Part model, mm, in its own coordinate system. Face numbers are marked on the shaded views. A direction names the side the tool comes from. Give positions to 0.01 mm unless a question says otherwise; leave off trailing zeros. Write each loop counter-clockwise with the first axis right and the second up, starting at its lowest first coordinate (ties: lowest second). Pieces come first, ordered by that corner, then holes. Notation, with made-up numbers: (89, 64.5) - (148, 64.5) arc R34 ccw to (148, 98.5) - close; hole circle Ø8 at (24, 34). An arc over 180 degrees is marked (long way). Answer as a JSON object with one key per item and string values. Group by question number.
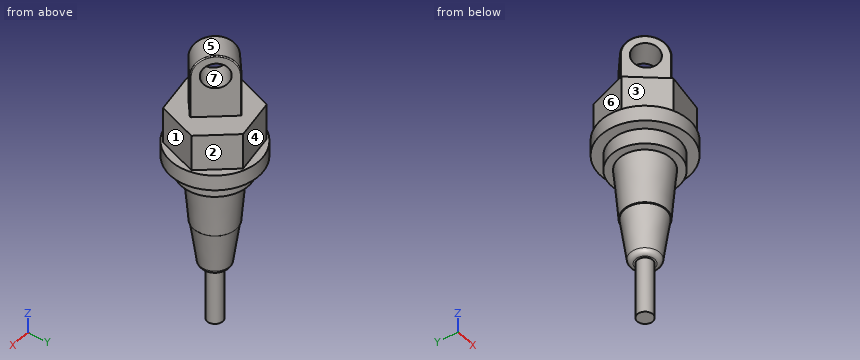
```python
from build123d import *

# Parameters (mm, degrees)
SKETCH_1_R      = 8.5
EXTRUDE_1_DEPTH = 3
EXTRUDE_2_DEPTH = 7
SKETCH_3_R      = 6.5
EXTRUDE_3_DEPTH = 3
SKETCH_4_R      = 5
EXTRUDE_4_DEPTH = 10
EXTRUDE_4_TAPER = 5
SKETCH_5_R      = 4
EXTRUDE_5_DEPTH = 9
EXTRUDE_5_TAPER = 8
FILLET_1_R      = 0.1
FILLET_2_R      = 1
SKETCH_7_R      = 2.5
EXTRUDE_6_DEPTH = 2.5
FILLET_3_R      = 0.2
SKETCH_8_R      = 1.5
EXTRUDE_7_DEPTH = 11


with BuildPart() as part:
    # 草图1 → 凸台-拉伸1 (new body)
    with BuildSketch(Plane.XY):
        with Locations((0, 6.282173928)):
            Circle(SKETCH_1_R)
    extrude(amount=EXTRUDE_1_DEPTH)

    # 草图2 → 凸台-拉伸2 (add)
    with BuildSketch(Plane.XY.offset(3)):
        Polygon((5.281387937, 0.163328057), (7.939769935, 7.796567113), (2.658381997, 13.915412984), (-5.281387937, 12.401019799), (-7.939769935, 4.767780743), (-2.658381997, -1.351065128), align=None)
    extrude(amount=EXTRUDE_2_DEPTH)

    # 草图3 → 凸台-拉伸3 (add)
    with BuildSketch(Plane(origin=(0, 0, 0), x_dir=(-1, 0, 0), z_dir=(0, 0, -1))):
        with Locations(Location((0, 6.282173928, 0), (0, 0, 180))):
            Circle(SKETCH_3_R)
    extrude(amount=EXTRUDE_3_DEPTH)

    # 草图4 → 凸台-拉伸4 (add)
    with BuildSketch(Plane(origin=(0, 0, -3), x_dir=(-1, 0, 0), z_dir=(0, 0, -1))):
        with Locations((0, 6.282173928)):
            Circle(SKETCH_4_R)
    extrude(amount=EXTRUDE_4_DEPTH, taper=EXTRUDE_4_TAPER)

    # 草图5 → 凸台-拉伸5 (add)
    with BuildSketch(Plane(origin=(0, 0, -13), x_dir=(-1, 0, 0), z_dir=(0, 0, -1))):
        with Locations((0, 6.282173928)):
            Circle(SKETCH_5_R)
    extrude(amount=EXTRUDE_5_DEPTH, taper=EXTRUDE_5_TAPER)

    # 圆角1
    fillet_1_edges = [part.edges().sort_by_distance(p)[0] for p in [
        (4.125113365, 6.282173928, -13),
    ]]
    fillet(fillet_1_edges, radius=FILLET_1_R)

    # 圆角2
    fillet_2_edges = [part.edges().sort_by_distance(p)[0] for p in [
        (2.735132488, 6.282173928, -22),
    ]]
    fillet(fillet_2_edges, radius=FILLET_2_R)

    # 草图7 → 凸台-拉伸6 (add, symmetric)
    with BuildSketch(Plane(origin=(3.107368239, 2.682077222, 0), x_dir=(0, 0, 1), z_dir=(-0.7570108522857268, -0.6534023029662793, 0))):
        with BuildLine():
            Line((10, 8.797125724), (18.23150741, 8.797125724))
            ThreePointArc((18.23150741, 8.797125724), (22.272959294, 4.755673839), (18.23150741, 0.714221955))
            Line((18.23150741, 0.714221955), (10, 0.714221955))
            Line((10, 0.714221955), (10, 8.797125724))
        make_face()
        with Locations(Location((18.23150741, 4.755673839, 0), (0, 0, 270))):
            Circle(SKETCH_7_R, mode=Mode.SUBTRACT)
    extrude(amount=EXTRUDE_6_DEPTH, both=True)

    # 圆角3
    fillet_3_edges = [part.edges().sort_by_distance(p)[0] for p in [
        (0.748166838, 1.589245235, 14.115753705),
        (-1.892527131, 4.648668171, 22.272959294),
        (-4.533221099, 7.708091106, 14.115753705),
        (4.533221099, 4.85625675, 14.115753705),
        (1.892527131, 7.915679685, 22.272959294),
        (-0.748166838, 10.975102621, 14.115753705),
    ]]
    fillet(fillet_3_edges, radius=FILLET_3_R)

    # 草图8 → 凸台-拉伸7 (add)
    with BuildSketch(Plane(origin=(0, 0, -22), x_dir=(-1, 0, 0), z_dir=(0, 0, -1))):
        with Locations((0, 6.282173928)):
            Circle(SKETCH_8_R)
    extrude(amount=EXTRUDE_7_DEPTH)


solid = part.part
```
1) Mould opens along X. For the marked faces 5, 6 and 7 say: pulls with the +X half, pulls with the -X half, needs draft (parallel to the pull), parting line crosses it, or undercut.
2) Band-saw the part on B-B (z = -11). List the corners of the cut face in (x, y), plus the area to 3 significant figures.
3) Band-saw the part on C-C (z = -18.5). List the corners of the cut face in (x, y), plus the area to 3 significant figures.
4) Probe line 1 (Z direction, x = -5.25, y = 12.75); line 2 (Z direction, x = 6.25, y = 8.75); line 3 (Y direction, x = 7.5, z = 1.5). List the from-to ranges inside material, lowest first.
5) Band-saw the part on A-A (x = 7). List the corners of the cut face in (y, z).
6) Drop flat-ended pins along their axis: P1, Ø4.5, axis at x = 0, y = 3, coming from the +Z side; P2, Ø2, axis at x = 3.5, z = 3.5, coming from the +Y side; P3, Ø2, axis at x = 0.5, y = 9, coming from the -Z side; P4, Ø1.5, axis at y = 10, z = -22.5, coming from the +X side. Give the stop position or say it passes through.
7) Which spindle directions (+Z, -Z, +X, -X, +Y, -Y) get a long thin tool onto all of the face, cutting with end or side? Do the marked faces 1, 2, 3 and 4. Say none if no direction does.
Verdict:
{
 "1": {"face 5": "parting line crosses it", "face 6": "pulls with the -X half", "face 7": "undercut"},
 "2": {"outline": "circle Ø8.6 at (0, 6.28)", "area": "58.1 mm2"},
 "3": {"outline": "circle Ø6.45 at (0, 6.28)", "area": "32.7 mm2"},
 "4": {"line 1": "0 to 3", "line 2": "0 to 10", "line 3": "2.28 to 10.28"},
 "5": {"outline": "(1.46, 0) - (11.1, 0) - (11.1, 3) - (8.89, 3) - (8.89, 10) - (5.1, 10) - (5.1, 3) - (1.46, 3) - close"},
 "6": {"P1": "z = 22.27", "P2": "y = 14.36", "P3": "z = -22", "P4": "through"},
 "7": {"face 1": "+Z, +X, -Y", "face 2": "+Z, +X, +Y", "face 3": "+Z, -X, -Y", "face 4": "+Z, -X, +Y"}
}
